Build history of the part. All positions in model axes, mm. Face numbers are marked on the shaded views. A direction names the side the tool comes from. Coordinates: 2 decimals unless noted, no trailing zeros. Loops run counter-clockwise (first coordinate to the right, second up) from the corner with the lowest first, then second, coordinate; pieces in that order, holes last. Notation, with made-up numbers: (-19, 78.5) - (20, 78.5) arc R25 ccw to (20, 106.5) - close; hole circle Ø4 at (31, 55.5). An arc over 180 degrees is marked (long way). One line per item, written item: value.
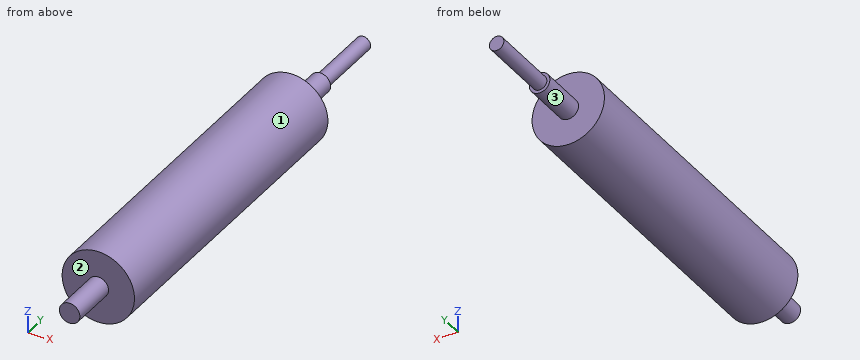
Autodesk Inventor part; units mm, degrees
ref_plane "YZ Plane" through (0, 0, 0) normal (1, 0, 0) x (0, 1, 0)
ref_plane "XZ Plane" through (0, 0, 0) normal (0, 1, 0) x (-1, 0, 0)
ref_plane "XY Plane" through (0, 0, 0) normal (0, 0, 1) x (1, 0, 0)
sketch "Sketch1" plane through (0, 0, 0) normal (0, 1, 0) x (-1, 0, 0)
  circle A0 centre (0, 0) radius 30
  dimension "d0" = 60
extrude "Extrusion1" add sketch "Sketch1" along normal mid plane 270
sketch "Sketch2" plane through (0, -135, 0) normal (0, -1, 0) x (1, 0, 0)
  circle A0 centre (0, 0) radius 8.5
  dimension "d3" = 17
extrude "Extrusion2" add sketch "Sketch2" along normal blind 40
sketch "Sketch3" plane through (0, 135, 0) normal (0, 1, 0) x (1, 0, 0)
  circle A0 centre (0, 0) radius 8.5
  circle A1 centre (0, 0) radius 8.5
  dimension "d6" = 17
extrude "Extrusion3" add sketch "Sketch3" along normal blind 100
sketch "Sketch4" plane through (0, 235, 0) normal (0, 1, 0) x (1, 0, 0)
  circle A0 centre (0, 0) radius 8.5
  circle A1 centre (0, 0) radius 6
  dimension "d9" = 12
extrude "Extrusion4" cut sketch "Sketch4" against normal blind 60
properties part number "HCMUTE-CDT23-TRUC_DAN" material "Stainless Steel"
Item 1: Drop flat-ended pins along their axis: P1, Ø1, axis at y = -127.5, z = -13.5, coming from the -X side; P2, Ø1.5, axis at x = 6, z = 3.5, coming from the +Y side; P3, Ø4, axis at x = 19.5, z = -11, coming from the +Y side. Give the stop position or say it passes through.
Check result:
P1: stops at x = -27.04
P2: stops at y = 175
P3: stops at y = 135
Item 2: Tool access for the marked faces 1, 2 and 3: list every direction of +Z, -Z, +X, -X, +Y, -Y with a clear straight run to the whole face (end or side of a thin tool).
Check result:
face 1: +Y, -Y
face 2: -Y
face 3: +Y
Item 3: Cut at D-D, the plane x = 23. Write the cut outline in (y, z), then the cut area to 3 significant figures.
Check result:
outline: (-135, -19.26) - (135, -19.26) - (135, 19.26) - (-135, 19.26) - close
area: 10,400 mm^2
Item 4: Cut at A-A, the plane x = 0. Write the cut outline in (y, z).
Check result:
outline: (-175, -8.5) - (-135, -8.5) - (-135, -30) - (135, -30) - (135, -8.5) - (175, -8.5) - (175, -6) - (235, -6) - (235, 6) - (175, 6) - (175, 8.5) - (135, 8.5) - (135, 30) - (-135, 30) - (-135, 8.5) - (-175, 8.5) - close
Item 5: Cut at C-C, the plane y = 121.5. Write the cut outline in (x, z), then the cut area to 3 significant figures.
Check result:
outline: circle Ø60 at (0, 0)
area: 2,830 mm^2
Item 6: Cut at B-B, the plane z = 0. Write the cut outline in (x, y), then the cut area to 3 significant figures.
Check result:
outline: (-30, -135) - (-8.5, -135) - (-8.5, -175) - (8.5, -175) - (8.5, -135) - (30, -135) - (30, 135) - (8.5, 135) - (8.5, 175) - (6, 175) - (6, 235) - (-6, 235) - (-6, 175) - (-8.5, 175) - (-8.5, 135) - (-30, 135) - close
area: 18,300 mm^2
Item 7: Probe probe 1 along Y at (x, z) = (7, 6); probe 2 along X at (y, z) = (-65, 1.5); probe 3 along Z at (x, y) = (-0.5, -140.5). List the from-to ranges inside material, lowest first. Write a range as from..to.
Check result:
probe 1: y = -135..135
probe 2: x = -29.96..29.96
probe 3: z = -8.49..8.49
